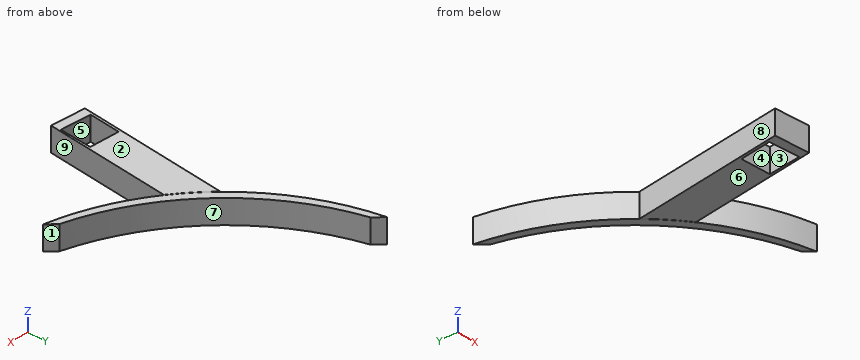
from build123d import *

# Parameters (mm, degrees)
BOSS_EXTRUDE1_DEPTH             = 10
SCALE1_SCALE                    = 0.5
BOSS_EXTRUDE2_REACH             = 46.064
BOSS_EXTRUDE2_END_RADIUS        = 47.489459432
SKETCH4_W                       = 5
SKETCH4_H                       = 7
BOSS_EXTRUDE2_DIRECTION_2_DEPTH = 20
CUT_EXTRUDE1_DEPTH              = 42.005284287


with BuildPart() as part:
    # Sketch1 → Boss-Extrude1 (new body)
    with BuildSketch(Plane.XY):
        with BuildLine():
            Line((40.984301278, -16.277292989), (37.448767372, -12.741759083))
            ThreePointArc((37.448767372, -12.741759083), (-4.964984169, 12.060025443), (-29.766768694, 54.473776984))
            Line((-29.766768694, 54.473776984), (-33.3023026, 58.00931089))
            ThreePointArc((-33.3023026, 58.00931089), (-7.365037029, 9.659972583), (40.984301278, -16.277292989))
        make_face()
    extrude(amount=BOSS_EXTRUDE1_DEPTH)


with BuildPart() as part_1:
    # Scale1: scaled about (-3.035293352, 13.98971626, 5)
    add(part.part.scale(SCALE1_SCALE).moved(Location((-1.517646676, 6.99485813, 2.5))))

    # Boss-Extrude2: up to this cylinder (the profile starts outside it)
    boss_extrude2_end = Plane(origin=(28.379953609, 45.404963221, 5.043467), z_dir=(0, 0, -1)) * Cylinder(BOSS_EXTRUDE2_END_RADIUS, 188.106918865, mode=Mode.PRIVATE)
    # Sketch4 → Boss-Extrude2 (add, up to the surface)
    with BuildSketch(Plane(origin=(7.010218182, 0.680511093, -0.258230649), x_dir=(0, 0, -1), z_dir=(0.08715574274766595, 0.9961946980917449, 0)), mode=Mode.PRIVATE) as boss_extrude2_sk1:
        with Locations((-5.301697823, 10.489820344)):
            Rectangle(SKETCH4_W, SKETCH4_H)
    boss_extrude2_tool1 = extrude(boss_extrude2_sk1.sketch, amount=BOSS_EXTRUDE2_REACH, mode=Mode.PRIVATE) - boss_extrude2_end
    add(boss_extrude2_tool1.solids().sort_by_distance((-3.439685, 1.594759, 5.043467))[0])

    # Sketch4 → Boss-Extrude2 direction 2 (add)
    with BuildSketch(Plane(origin=(7.010218182, 0.680511093, -0.258230649), x_dir=(0, 0, -1), z_dir=(0.08715574274766595, 0.9961946980917449, 0))):
        with Locations((-5.301697823, 10.489820344)):
            Rectangle(SKETCH4_W, SKETCH4_H)
    extrude(amount=-BOSS_EXTRUDE2_DIRECTION_2_DEPTH)

    # Sketch10 → Cut-Extrude1 (cut, through all)
    with BuildSketch(Plane.XY.offset(7.543467174)):
        Polygon((-8.004005245, -16.209052666), (-7.451990048, -9.899490092), (-1.451990048, -10.245322297), (-1.874415312, -16.745322297), align=None)
    extrude(amount=-CUT_EXTRUDE1_DEPTH, mode=Mode.SUBTRACT)


solid = part_1.part
Check sheet for the modelled part. Datum: model origin and axes. Units: mm. Face numbers are marked on the shaded views. A direction names the side the tool comes from. Coordinates: 2 decimals unless noted, no trailing zeros. Write each loop counter-clockwise with the first axis right and the second up, starting at its lowest first coordinate (ties: lowest second). Pieces come first, ordered by that corner, then holes.
Item 1: Access from +Z, -Z, +X, -X, +Y, -Y to the whole of each face (thin tool, end or side, straight path). Record for the marked faces 5, 6, 7, 8 and 9.
Numbers:
face 5: +Z, -Z
face 6: -Z, -X, -Y
face 7: +Z, -Z, +X, +Y
face 8: +Z, -Z, -X
face 9: +Z, -Z, -Y
Item 2: Cross-section at B-B on y = -13.5. Record the boundary of the cut face in (x, z), then the cut area to 3 significant figures.
Numbers:
outline: (-8.27, 2.54) - (-7.77, 2.54) - (-7.77, 7.54) - (-8.27, 7.54) - close; (-1.66, 2.54) - (-1.25, 2.54) - (-1.25, 7.54) - (-1.66, 7.54) - close
area: 4.62 mm2
Item 3: Cross-section at C-C on x = 0. Record the boundary of the cut face in (y, z).
Numbers:
outline: (0.75, 2.54) - (7.33, 2.54) - (7.33, 2.5) - (9.45, 2.5) - (9.45, 7.5) - (7.33, 7.5) - (7.33, 7.54) - (0.75, 7.54) - close
Item 4: Cross-section at A-A on z = 5.4. Record the boundary of the cut face in (x, y), then the cut area to 3 significant figures.
Numbers:
outline: (-18.17, 36) arc R47.49 ccw to (-5.99, 12.63) - (-8.67, -18.02) - (-1.7, -18.63) - (0.54, 6.93) arc R47.49 ccw to (18.97, -1.14) - (17.21, 0.62) arc R48.46 cw to (-16.4, 34.23) - close; hole (-8, -16.21) - (-1.87, -16.75) - (-1.45, -10.25) - (-7.45, -9.9) - close
area: 240 mm2
Item 5: Mould release check, pull along X, two halves, no side actions. Record for the marked faces 1, 2, 3 and 4: released by +X, released by -X, zero draft, split by the parting line, or undercut.
Numbers:
face 1: released by +X
face 2: zero draft
face 3: undercut
face 4: undercut
Item 6: Depth check by flat-ended pin: pin 1 Ø2 at (x, z) = (6.5, 3) entering from +Y; pin 2 Ø3 at (y, z) = (-12.5, 4.5) entering from +X; pin 3 Ø3 at (x, z) = (11, 5.5) entering from +Y; pin 4 Ø4 at (x, y) = (8.5, 1) entering from -Z. Enter the tip coordinate at first touch or a pass-through.
Numbers:
pin 1: stops at y = 5.64
pin 2: stops at x = -1.03
pin 3: stops at y = 3.51
pin 4: stops at z = 2.5
Item 7: Cross-section at D-D on y = 3. Record the boundary of the cut face in (x, z), then the cut area to 3 significant figures.
Numbers:
outline: (-6.83, 2.54) - (0.2, 2.54) - (0.2, 7.54) - (-6.83, 7.54) - close; (7, 2.5) - (10.6, 2.5) - (10.6, 7.5) - (7, 7.5) - close
area: 53.1 mm2
Item 8: Scan lines: probe 1 along X at (y, z) = (2.5, 4.35); probe 2 along X at (y, z) = (-14, 3.6); probe 3 along Y at (x, z) = (-4.5, 3.75). Record each from-to range of solid material in increasing order.
Numbers:
probe 1: x = -6.87 to 0.15, 8.02 to 11.77
probe 2: x = -8.32 to -7.81, -1.7 to -1.29
probe 3: y = -18.39 to -16.52, -10.07 to 13.53
